Read the model definition and answer for the solid it produces. Units are mm, in the model's axes. Face numbers are marked on the shaded views. A direction names the side the tool comes from. Give positions to 0.01 mm unless a question says otherwise; leave off trailing zeros. Write each loop counter-clockwise with the first axis right and the second up, starting at its lowest first coordinate (ties: lowest second). Pieces come first, ordered by that corner, then holes. Notation, with made-up numbers: (-5, 67) -> (27, 67) arc R14 ccw to (27, 84) -> close; hole circle Ø1 at (6.25, -4.75). An arc over 180 degrees is marked (long way). Write item = value, one per line.
from build123d import *

# Parameters (mm, degrees)
SKETCH1_R          = 19
EXTRUDE1_DEPTH     = 3
SKETCH2_R          = 12.75
EXTRUDE2_DEPTH     = 51
EXTRUDE3_START     = -26
EXTRUDE3_OUTLINE_R = 5
EXTRUDE3_DEPTH     = 26
EXTRUDE5_START     = -28
EXTRUDE5_OUTLINE_R = 3
EXTRUDE5_DEPTH     = 28
CHAMFER1_SIZE      = 1.57
SCALE1_SCALE       = 0.5


# Read off the part's stored shape, not the designer's step: Extrude3, Extrude5
with BuildPart() as part:
    # Sketch1 → Extrude1 (new body)
    with BuildSketch(Plane.XY):
        Circle(SKETCH1_R)
    extrude(amount=EXTRUDE1_DEPTH)

    # Sketch2 → Extrude2 (add)
    with BuildSketch(Plane(origin=(0, 0, 0), x_dir=(-1, 0, 0), z_dir=(0, 0, -1))):
        with Locations(Location((0, 0, 0), (0, 0, 180))):
            Circle(SKETCH2_R)
    extrude(amount=EXTRUDE2_DEPTH)

    # Extrude3 outline → Extrude3 (cut)
    with BuildSketch(Plane.XY.offset(3).offset(EXTRUDE3_START)):
        Circle(EXTRUDE3_OUTLINE_R)
    extrude(amount=EXTRUDE3_DEPTH, mode=Mode.SUBTRACT)

    # Extrude5 outline → Extrude5 (cut)
    with BuildSketch(Plane(origin=(0, 0, -51), x_dir=(-1, 0, 0), z_dir=(0, 0, -1)).offset(EXTRUDE5_START)):
        Circle(EXTRUDE5_OUTLINE_R)
    extrude(amount=EXTRUDE5_DEPTH, mode=Mode.SUBTRACT)

    # Chamfer1
    chamfer1_edges = [part.edges().sort_by_distance(p)[0] for p in [
        (3, 0, -23),
    ]]
    chamfer(chamfer1_edges, length=CHAMFER1_SIZE)


with BuildPart() as part_1:
    # Scale1: scaled about (0, 0, 0)
    add(part.part.scale(SCALE1_SCALE))


solid = part_1.part
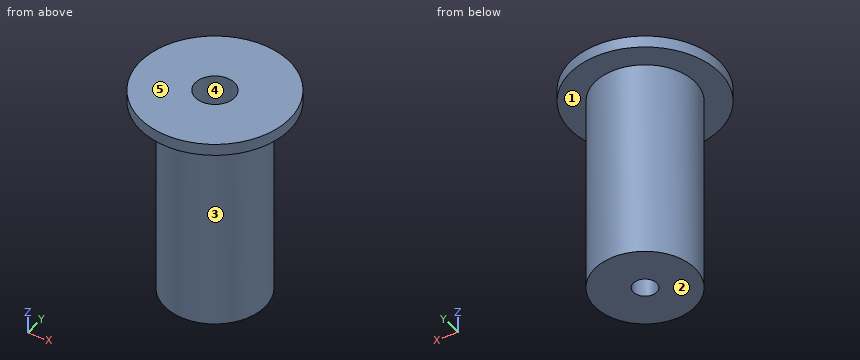
(1) The part is cut by section D-D on x = -4. Determine the outline of the cut face in (y, z), plus the area to 3 significant figures.
Checks:
outline = (-8.62, 0) -> (-4.96, 0) -> (-4.96, -25.5) -> (4.96, -25.5) -> (4.96, 0) -> (8.62, 0) -> (8.62, 1.5) -> (-8.62, 1.5) -> close
area = 279 mm²
(2) The part is cut by section C-C on z = -18. Determine the outline of the cut face in (x, y) (3 decimals).
Checks:
outline = circle Ø12.75 at (0, 0); hole circle Ø3 at (0, 0)
(3) A tool of negligible diameter and unlimited length cuts with its end or side. For the marked faces 1 and 2, from which of +Z, -Z, +X, -X, +Y, -Y can it reach the whole face along a straight path? Write none if from no direction.
Checks:
face_1 = -Z
face_2 = -Z, +X, -X, +Y, -Y
(4) For a pull along Y with two mould halves and no side action, classify the marked faces 3, 4 and 5 as released by +Y, released by -Y, zero draft, split by the parting line, or undercut.
Checks:
face_3 = split by the parting line
face_4 = undercut
face_5 = zero draft
(5) The part is cut by section A-A on y = 0. Determine the outline of the cut face in (x, z) (3 decimals), plus the area to 3 significant figures.
Checks:
outline = (-9.5, 0) -> (-6.375, 0) -> (-6.375, -25.5) -> (-1.5, -25.5) -> (-1.5, -12.285) -> (-2.285, -11.5) -> (-2.5, -11.5) -> (-2.5, 1.5) -> (-9.5, 1.5) -> close; (1.5, -25.5) -> (6.375, -25.5) -> (6.375, 0) -> (9.5, 0) -> (9.5, 1.5) -> (2.5, 1.5) -> (2.5, -11.5) -> (2.285, -11.5) -> (1.5, -12.285) -> close
area = 246 mm²
(6) Given P1, Ø2, axis at x = -4.5, z = -19.5, coming from the +Y side; P2, Ø8, axis at x = 5, z = -2.5, coming from the +Y side; P3, Ø1.5, axis at x = -2, z = -14, coming from the -Y side, each flat-ended and moving along its own axis, determine where each tip first touches the part or whether it passes through.
Checks:
P1 = 5.33
P2 = 9.31
P3 = -6.25
(7) Consider L1, parallel to Y at x = 0, z = -6 (3 decimals); L2, parallel to Y at x = 0, z = -19.5 (3 decimals); L3, parallel to Z at x = 3, y = 7.75. Determine where each line is inside the solid, lowest interval first.
Checks:
L1 = -6.375 to -2.5, 2.5 to 6.375
L2 = -6.375 to -1.5, 1.5 to 6.375
L3 = 0 to 1.5
